Geometry: see drawing. Coordinates: mm, zero at the bounding-box minimum. Give positions to 0.01 mm unless a question says otherwise; leave off trailing zeros. Order: outer loops, then holes, each group sorted by start corner. A loop starts at its lowest first (then second) coordinate and runs counter-clockwise, first axis right, second up. Notation, with made-up numbers: (-14.75, -13.5) - (36.25, -13.5) arc R23 ccw to (36.25, 5.5) - close; hole circle Ø10 at (55.5, 70.25). An arc over 180 degrees is marked (long way). One line per item, written item: value.
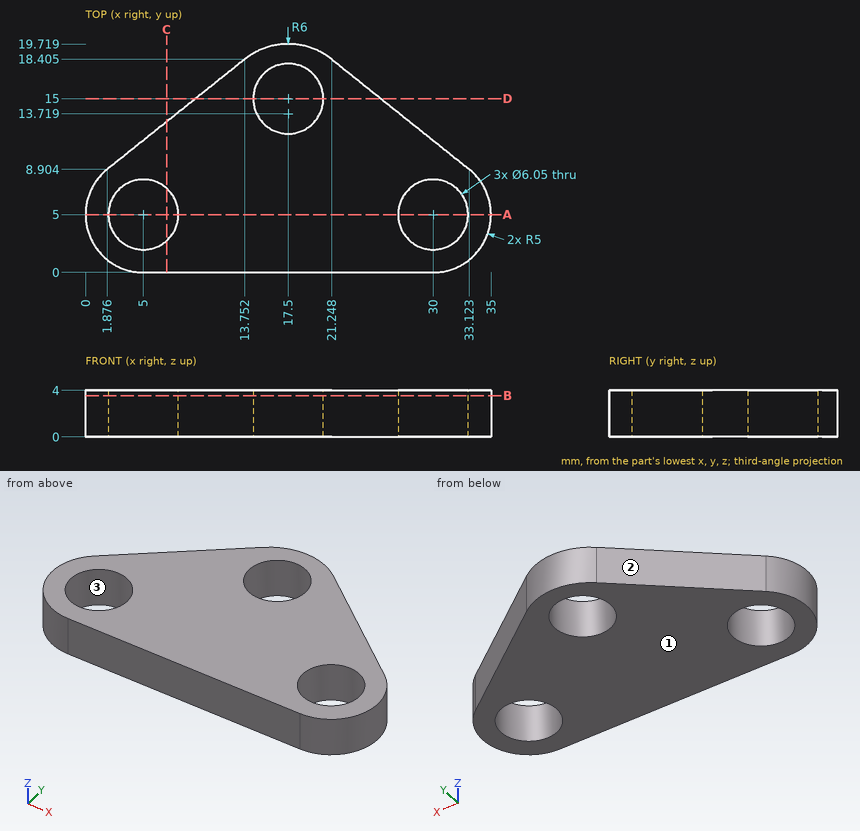
1) Section A-A, the plane y = 5. Return loops of the section in (x, z) (1 decimal).
Answers below:
outline: (0, 0) - (2, 0) - (2, 4) - (0, 4) - close; (8, 0) - (27, 0) - (27, 4) - (8, 4) - close; (33, 0) - (35, 0) - (35, 4) - (33, 4) - close
2) Mould query, pull axis X, two halves, no side actions, for the marked faces 1, 2 and 3. Classes: released by +X, released by -X, zero draft, split by the parting line, or undercut.
Answers below:
face 1: zero draft
face 2: released by -X
face 3: undercut
3) Section D-D, the plane y = 15. Return loops of the section in (x, z) (1 decimal).
Answers below:
outline: (9.5, 0) - (14.5, 0) - (14.5, 4) - (9.5, 4) - close; (20.5, 0) - (25.5, 0) - (25.5, 4) - (20.5, 4) - close
4) Material intervals for line 1 along Y through (x, z) = (27.5, 2.2) (1 decimal); line 2 along X through (y, z) = (3, 1.8) (1 decimal); line 3 along Y through (x, z) = (19.5, 3.55) (1 decimal), sorted ascending.
Answers below:
line 1: 0 to 3.3, 6.7 to 13.4
line 2: 0.4 to 2.7, 7.3 to 27.7, 32.3 to 34.6
line 3: 0 to 12.7, 17.3 to 19.4
5) Section C-C, the plane x = 7. Return loops of the section in (y, z).
Answers below:
outline: (0, 0) - (2.73, 0) - (2.73, 4) - (0, 4) - close; (7.27, 0) - (13, 0) - (13, 4) - (7.27, 4) - close
6) First-contact query: pin 1 (1.5 mm diameter, centred on x = 11, z = 3, fed in from +Y); pin 2 (9.5 mm diameter, centred on x = 17.5, y = 15, fed in from +Z); pin 3 (1 mm diameter, centred on x = 31, z = 3.5, fed in from -Y) (1 decimal). Flat tips, straight axial feed; report the tip coordinate or a pass-through.
Answers below:
pin 1: y = 16.8
pin 2: z = 4
pin 3: y = 0
7) Section B-B, the plane z = 3.55. Count the separate pieces of the cut face and the enclosed holes in it, then the cut area to 3 significant figures.
Answers below:
separate pieces: 1
enclosed holes: 3
area: 401 mm^2
